Design review of the part built by this model. Coordinates are the model's own, in mm. Face numbers are marked on the shaded views. Coordinates: 2 decimals unless noted, no trailing zeros. Loops run counter-clockwise (first coordinate to the right, second up) from the corner with the lowest first, then second, coordinate; pieces in that order, holes last. Notation, with made-up numbers: M 35,-28.5 L 87,-28.5 A17 cw 87,3.5 Z; hole C -14,-16.5 d7. An arc over 180 degrees is marked long. Answer as a JSON object with one key per item and string values. Group by question number.
1. Draft analysis for pull direction Y (two halves, no side actions). For the marked faces 1, 2 and 3, state which applies: +Y half, -Y half, draft (parallel to the pull), parting line (faces both ways), or undercut.
2. Insertion check: pin 1 (2.5 mm diameter, centred on x = -5.5, y = 2, fed in from -Z). The pin has a flat end and moves straight along its axis. Give the tip position at first contact, or say it passes through.
3. To check wall thickness, follow probe 1 along Y at (x, z) = (1, 4.6); probe 2 along Y at (x, z) = (0.5, 1.15); probe 3 along Y at (x, z) = (-12, 3.2). State the ranges of each line that lie inside material, in increasing order.
4. Consider section B-B (x = 17). State the section outline as (y, z) points.
5. Consider section C-C (y = -4.25). State the section outline as (x, z) points.
6. Consider section D-D (y = 4). State the section outline as (x, z) points.
7. Consider section A-A (z = 3.15). State the section outline as (x, y) points, then the cut area to 3 significant figures.
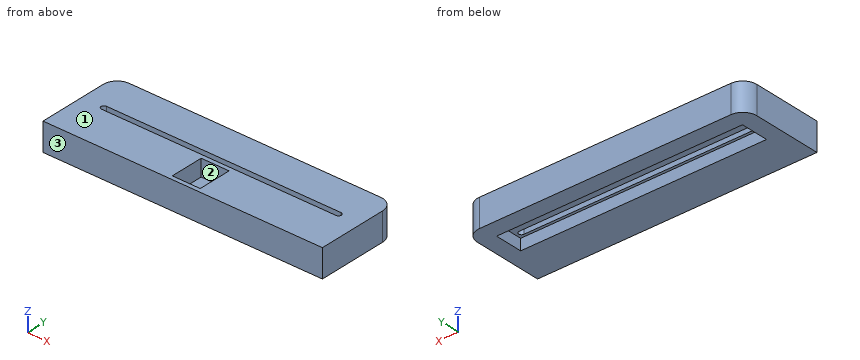
from build123d import *

# Parameters (mm, degrees)
CROQUIS1_W              = 50
CROQUIS1_H              = 15
CROQUIS1_W_2            = 44
CROQUIS1_H_2            = 5
SALIENTE_EXTRUIR1_DEPTH = 5
CROQUIS1_4_W            = 44
CROQUIS1_4_H            = 5
CORTAR_EXTRUIR1_DEPTH   = 2
REDONDEO1_R             = 2.5
CORTAR_EXTRUIR2_DEPTH   = 27.272609311
CROQUIS3_W              = 5
CROQUIS3_H              = 6
CORTAR_EXTRUIR3_DEPTH   = 3


with BuildPart() as part:
    # Croquis1 → Saliente-Extruir1 (new body)
    with BuildSketch(Plane.XY):
        Rectangle(CROQUIS1_W, CROQUIS1_H)
        with Locations((0, 2)):
            Rectangle(CROQUIS1_W_2, CROQUIS1_H_2, mode=Mode.SUBTRACT)
        with Locations((0, 2)):
            Rectangle(CROQUIS1_W_2, CROQUIS1_H_2)
    extrude(amount=SALIENTE_EXTRUIR1_DEPTH)

    # Croquis1_4 → Cortar-Extruir1 (cut)
    with BuildSketch(Plane.XY):
        with Locations((0, 2)):
            Rectangle(CROQUIS1_4_W, CROQUIS1_4_H)
    extrude(amount=CORTAR_EXTRUIR1_DEPTH, mode=Mode.SUBTRACT)

    # Redondeo1
    redondeo1_edges = [part.edges().sort_by_distance(p)[0] for p in [
        (-25, 7.5, 2.5),
        (25, 7.5, 2.5),
    ]]
    fillet(redondeo1_edges, radius=REDONDEO1_R)

    # Croquis2 → Cortar-Extruir2 (cut, through all)
    with BuildSketch(Plane(origin=(0, 0, 2), x_dir=(-1, 0, 0), z_dir=(0, 0, -1))):
        with BuildLine():
            Line((-21, 1), (21, 1))
            ThreePointArc((21, 1), (21.5, 0.5), (21, 0))
            Line((21, 0), (-21, 0))
            ThreePointArc((-21, 0), (-21.5, 0.5), (-21, 1))
        make_face()
    extrude(amount=-CORTAR_EXTRUIR2_DEPTH, mode=Mode.SUBTRACT)

    # Croquis3 → Cortar-Extruir3 (cut)
    with BuildSketch(Plane.XY.offset(5)):
        with Locations((0, -3.760126058)):
            Rectangle(CROQUIS3_W, CROQUIS3_H)
    extrude(amount=-CORTAR_EXTRUIR3_DEPTH, mode=Mode.SUBTRACT)


solid = part.part
Findings below:
{
 "1": {"face 1": "draft", "face 2": "undercut", "face 3": "-Y half"},
 "2": {"pin 1": "stops at z = 2"},
 "3": {"probe 1": "y = -7.5 to -6.76, -0.76 to 0, 1 to 7.5", "probe 2": "y = -7.5 to -0.5, 4.5 to 7.5", "probe 3": "y = -7.5 to 0, 1 to 7.5"},
 "4": {"outline": "M -7.5,0 L -0.5,0 L -0.5,2 L 0,2 L 0,5 L -7.5,5 Z; M 1,2 L 4.5,2 L 4.5,0 L 7.5,0 L 7.5,5 L 1,5 Z"},
 "5": {"outline": "M -25,0 L 25,0 L 25,5 L 2.5,5 L 2.5,2 L -2.5,2 L -2.5,5 L -25,5 Z"},
 "6": {"outline": "M -25,0 L -22,0 L -22,2 L 22,2 L 22,0 L 25,0 L 25,5 L -25,5 Z"},
 "7": {"outline": "M -25,-7.5 L 25,-7.5 L 25,5 A2.5 ccw 22.5,7.5 L -22.5,7.5 A2.5 ccw -25,5 Z; hole M -21,0 L 21,0 A0.5 ccw 21,1 L -21,1 A0.5 ccw Z; hole M -2.5,-6.76 L 2.5,-6.76 L 2.5,-0.76 L -2.5,-0.76 Z", "area": "675 mm^2"}
}
